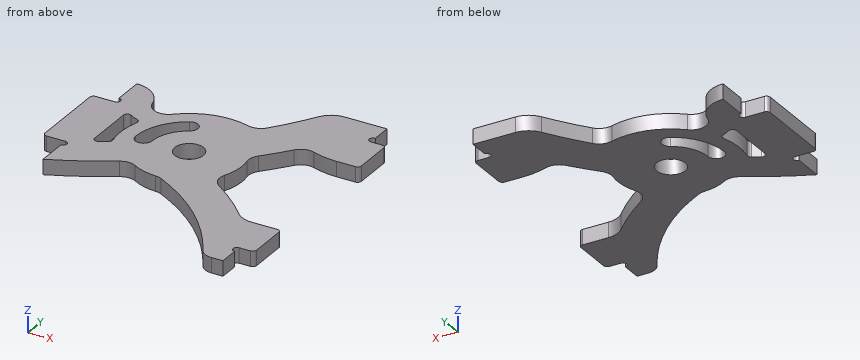
from build123d import *

# Parameters (mm, degrees)
BOSS_EXTRUDE1_DEPTH        = 2
M3_5_CLEARANCE_HOLE1_D     = 3.8
M3_5_CLEARANCE_HOLE1_DEPTH = 2


with BuildPart() as part:
    # Sketch1 → Boss-Extrude1 (new body)
    with BuildSketch(Plane.XY):
        with BuildLine():
            Line((18.63883017, -16.482761143), (18.63883017, -11.482761143))
            ThreePointArc((18.63883017, -11.482761143), (18.492383561, -11.129207753), (18.13883017, -10.982761143))
            Line((18.13883017, -10.982761143), (14.726824149, -10.982761143))
            ThreePointArc((14.726824149, -10.982761143), (13.539431255, -10.737774413), (12.545968697, -10.042826553))
            ThreePointArc((12.545968697, -10.042826553), (9.927684451, -7.539157578), (7.068753945, -5.314233513))
            ThreePointArc((7.068753945, -5.314233513), (6.287636427, -4.208593434), (6.389660154, -2.858713543))
            ThreePointArc((6.389660154, -2.858713543), (6.954343162, -0.798192452), (6.871191626, 1.336684568))
            ThreePointArc((6.871191626, 1.336684568), (6.905834234, 2.248382718), (7.341806065, 3.049832772))
            ThreePointArc((7.341806065, 3.049832772), (8.751272055, 4.692211544), (10.096999644, 6.387209969))
            ThreePointArc((10.096999644, 6.387209969), (11.122804542, 7.092577212), (12.367138803, 7.054486744))
            ThreePointArc((12.367138803, 7.054486744), (13.978037739, 6.625408008), (15.63883017, 6.480935011))
            Line((15.63883017, 6.480935011), (18.13883017, 6.480935011))
            ThreePointArc((18.13883017, 6.480935011), (18.492383561, 6.62738162), (18.63883017, 6.980935011))
            Line((18.63883017, 6.980935011), (18.63883017, 11.980935011))
            ThreePointArc((18.63883017, 11.980935011), (18.492383561, 12.334488401), (18.13883017, 12.480935011))
            Line((18.13883017, 12.480935011), (16.63883017, 12.480935011))
            ThreePointArc((16.63883017, 12.480935011), (16.13883017, 12.980935011), (16.63883017, 13.480935011))
            Line((16.63883017, 13.480935011), (16.63883017, 16.099008984))
            Line((16.63883017, 16.099008984), (11.035994897, 16.099008984))
            ThreePointArc((11.035994897, 16.099008984), (9.559562701, 15.710550285), (8.465485791, 14.645774297))
            ThreePointArc((8.465485791, 14.645774297), (6.726327278, 11.952270464), (4.820305649, 9.37414774))
            ThreePointArc((4.820305649, 9.37414774), (3.846646619, 8.704308056), (2.664831641, 8.701073056))
            ThreePointArc((2.664831641, 8.701073056), (-2.003730385, 8.876658411), (-6.144167501, 6.712615415))
            ThreePointArc((-6.144167501, 6.712615415), (-8.103077659, 6.282745016), (-9.450079267, 7.768579541))
            ThreePointArc((-9.450079267, 7.768579541), (-10.84668059, 10.040750561), (-13.36116983, 10.92990761))
            Line((-13.36116983, 10.92990761), (-13.36116983, 6.92990761))
            ThreePointArc((-13.36116983, 6.92990761), (-12.86116983, 6.42990761), (-13.36116983, 5.92990761))
            Line((-13.36116983, 5.92990761), (-15.86116983, 5.92990761))
            ThreePointArc((-15.86116983, 5.92990761), (-16.21472322, 5.783461001), (-16.36116983, 5.42990761))
            Line((-16.36116983, 5.42990761), (-16.36116983, -4.57009239))
            ThreePointArc((-16.36116983, -4.57009239), (-16.21472322, -4.92364578), (-15.86116983, -5.07009239))
            Line((-15.86116983, -5.07009239), (-13.36116983, -5.07009239))
            ThreePointArc((-13.36116983, -5.07009239), (-12.86116983, -5.57009239), (-13.36116983, -6.07009239))
            Line((-13.36116983, -6.07009239), (-13.36116983, -10.07009239))
            ThreePointArc((-13.36116983, -10.07009239), (-9.424252929, -8.211858727), (-5.645907876, -6.049347295))
            ThreePointArc((-5.645907876, -6.049347295), (-4.609540233, -5.744803026), (-3.565955999, -6.023616672))
            ThreePointArc((-3.565955999, -6.023616672), (-1.987644312, -6.711875303), (-0.289069284, -6.994028807))
            ThreePointArc((-0.289069284, -6.994028807), (0.134843139, -7.057521972), (0.535490188, -7.209886886))
            ThreePointArc((0.535490188, -7.209886886), (7.881477412, -12.437026609), (13.387941825, -19.576029874))
            ThreePointArc((13.387941825, -19.576029874), (14.121752395, -20.325710404), (15.134079043, -20.600835116))
            Line((15.134079043, -20.600835116), (16.63883017, -20.600835116))
            Line((16.63883017, -20.600835116), (16.63883017, -17.982761143))
            ThreePointArc((16.63883017, -17.982761143), (16.13883017, -17.482761143), (16.63883017, -16.982761143))
            Line((16.63883017, -16.982761143), (18.13883017, -16.982761143))
            ThreePointArc((18.13883017, -16.982761143), (18.492383561, -16.836314534), (18.63883017, -16.482761143))
        make_face()
        with BuildLine():
            Line((-10.86116983, -2.746889398), (-10.86116983, 3.698246713))
            ThreePointArc((-10.86116983, 3.698246713), (-10.599535477, 4.13777125), (-10.088442557, 4.117316916))
            ThreePointArc((-10.088442557, 4.117316916), (-9.528608488, 3.802221602), (-8.932994407, 3.561507855))
            ThreePointArc((-8.932994407, 3.561507855), (-8.642555945, 3.309647034), (-8.616730153, 2.926082957))
            ThreePointArc((-8.616730153, 2.926082957), (-9.089130193, 0.444648546), (-8.861194309, -2.071046938))
            ThreePointArc((-8.861194309, -2.071046938), (-8.88986137, -2.384945686), (-9.100629521, -2.619319341))
            ThreePointArc((-9.100629521, -2.619319341), (-9.610484862, -2.905923033), (-10.123517324, -3.186799942))
            ThreePointArc((-10.123517324, -3.186799942), (-10.617269173, -3.176322893), (-10.86116983, -2.746889398))
        make_face(mode=Mode.SUBTRACT)
        with BuildLine():
            ThreePointArc((-3.55, 6.148780367), (-6.148780367, 3.55), (-7.1, 0))
            ThreePointArc((-7.1, 0), (-6, -1.1), (-4.9, 0))
            ThreePointArc((-4.9, 0), (-4.243524479, 2.45), (-2.45, 4.243524479))
            ThreePointArc((-2.45, 4.243524479), (-2.047372056, 5.746152423), (-3.55, 6.148780367))
        make_face(mode=Mode.SUBTRACT)
    extrude(amount=BOSS_EXTRUDE1_DEPTH)

    # M3.5 Clearance Hole1
    with Locations(Plane(origin=(0, 0, 0), x_dir=(-1, 0, 0), z_dir=(0, 0, -1))):
        with Locations((0, 0)):
            Hole(M3_5_CLEARANCE_HOLE1_D / 2, depth=M3_5_CLEARANCE_HOLE1_DEPTH)


solid = part.part
Read the model definition and answer for the solid it produces. Units are mm, in the model's axes. Coordinates: 2 decimals unless noted, no trailing zeros. Loops run counter-clockwise (first coordinate to the right, second up) from the corner with the lowest first, then second, coordinate; pieces in that order, holes last.
Q1. Consider probe 1 along X at (y, z) = (-1, 1.2); probe 2 along X at (y, z) = (-1.5, 0.1); probe 3 along Y at (x, z) = (-13, 0.3). Determine where each line is inside the solid, lowest interval first.
Q2. The part is cut by section C-C on y = 2.5. Write down the section's boundary in (x, z).
Q3. The part is cut by section B-B on x = -3. Write down the section's boundary in (y, z), and give its area (3 significant figures).
Q4. The part is cut by section D-D on z = 0.7. Give the number of separate pieces and of enclosed holes in the cut face, and give its area (3 significant figures).
Q5. Each of these flat-tipped pins is pushed along its axis until it touches: pin 1 Ø0.8 at (x, z) = (17.5, 0.5) entering from -Y; pin 2 Ø2.5 at (x, y) = (0, 0) entering from -Z; pin 3 Ø1 at (x, z) = (-1, 0.5) entering from +Y; pin 4 Ø1 at (y, z) = (-10, 1) entering from -X. Where does it stop, or does it pass through?
Q6. The part is cut by section A-A on y = 10. Write down the section's boundary in (x, z), and give its area (3 significant figures).
Results below:
1. probe 1: x = -16.36 to -10.86, -9.04 to -6.46, -5.54 to -1.62, 1.62 to 6.93
1. probe 2: x = -16.36 to -10.86, -8.98 to -1.17, 1.17 to 6.84
1. probe 3: y = -9.92 to -5.92, -5.22 to 6.08, 6.78 to 10.91
2. outline: (-16.36, 0) - (-10.86, 0) - (-10.86, 2) - (-16.36, 2) - close; (-8.75, 0) - (-6.65, 0) - (-6.65, 2) - (-8.75, 2) - close; (-4.21, 0) - (6.99, 0) - (6.99, 2) - (-4.21, 2) - close
3. outline: (-6.32, 0) - (3.87, 0) - (3.87, 2) - (-6.32, 2) - close; (6.3, 0) - (8.59, 0) - (8.59, 2) - (6.3, 2) - close
3. area: 25.0 mm2
4. separate pieces: 1
4. enclosed holes: 3
4. area: 521 mm2
5. pin 1: stops at y = -16.98
5. pin 2: passes through
5. pin 3: stops at y = 9.09
5. pin 4: stops at x = -13.36
6. outline: (-13.36, 0) - (-10.8, 0) - (-10.8, 2) - (-13.36, 2) - close; (5.31, 0) - (18.64, 0) - (18.64, 2) - (5.31, 2) - close
6. area: 31.8 mm2
